The listing builds one solid part. Answer for the finished solid, in the listing's coordinates (mm). Give positions to 0.01 mm unless a question says otherwise; leave off trailing zeros. Write each loop counter-clockwise with the first axis right and the second up, starting at its lowest first coordinate (ties: lowest second). Pieces come first, ordered by that corner, then holes. Notation, with made-up numbers: M 36,-1.75 L 79,-1.75 A6 ccw 79,4.25 Z; hole C -21,-12.5 d8. An arc over 180 degrees is marked long. Return JSON: item names as keys, results as strings.
from build123d import *

# Parameters (mm, degrees)
FILLET_R = 1


with BuildPart() as con001:
    # Cone001 → Cone001 (revolve)
    with BuildSketch(Plane(origin=(0, 0, 1), x_dir=(1, 0, 0), z_dir=(0, -1, 0))):
        Polygon((0, 0), (13, 0), (23, 70), (0, 70), align=None)
    revolve(axis=Axis((0, 0, 1), (0, 0, 1)))


with BuildPart() as fillet_body:
    # Cone → Cone (revolve)
    with BuildSketch(Plane.XZ):
        Polygon((0, 0), (15, 0), (25, 70), (0, 70), align=None)
    revolve(axis=Axis((0, 0, 0), (0, 0, 1)))

    # Cut: cut Con001
    add(con001.part, mode=Mode.SUBTRACT)

    # Fillet
    fillet_edges = [fillet_body.edges().sort_by_distance(p)[0] for p in [
        (-22.857143, 0, 70),
    ]]
    fillet(fillet_edges, radius=FILLET_R)


solid = fillet_body.part
Item 1: Find the intervals of material crossed by line 1 (Z direction, x = -10.5, y = 2.5); line 2 (X direction, y = -6, z = 14.5); line 3 (Y direction, x = 6, z = 5), in increasing order.
Geometry results:
{"line 1": "z = 0 to 1", "line 2": "x = -15.98 to -13.67, 13.67 to 15.98", "line 3": "y = -14.52 to -12.17, 12.17 to 14.52"}
Item 2: A cutting plane is placed at C-C, the plane z = 9. Write down the section's boundary in (x, y), plus the area to 3 significant figures.
Geometry results:
{"outline": "C 0,0 d32.57; hole C 0,0 d28.29", "area": "205 mm2"}
Item 3: A cutting plane is placed at D-D, the plane z = 30. Write down the section's boundary in (x, y).
Geometry results:
{"outline": "C 0,0 d38.57; hole C 0,0 d34.29"}
Item 4: Determine the mould class of faces 1 (the flat face through (15, 19, 70)), 2 (the conical face through (-16, -12, 35)), 3 (the flat face through (0, 0, 1)) for opening direction Y: +Y half, -Y half, draft (parallel to the pull), parting line (faces both ways), or undercut.
Geometry results:
{"face 1": "draft", "face 2": "parting line", "face 3": "undercut"}
Item 5: Given pin 1 Ø3 at (x, z) = (7, 42) entering from +Y; pin 2 Ø5 at (x, z) = (9, 41) entering from -Y; pin 3 Ø3 at (y, z) = (-9.5, 12) entering from -X, each flat-ended and moving along its own axis, determine where each tip first touches the part or whether it passes through.
Geometry results:
{"pin 1": "stops at y = 20.32", "pin 2": "stops at y = -19.9", "pin 3": "stops at x = -14.71"}
Item 6: A cutting plane is placed at A-A, the plane y = 0. Write down the section's boundary in (x, z), plus the area to 3 significant figures.
Geometry results:
{"outline": "M -25,70 L -15,0 L 15,0 L 25,70 L 23.72,70 A1 ccw 22.73,69.14 L 13,1 L -13,1 L -22.73,69.14 A1 ccw -23.72,70 Z", "area": "326 mm2"}
